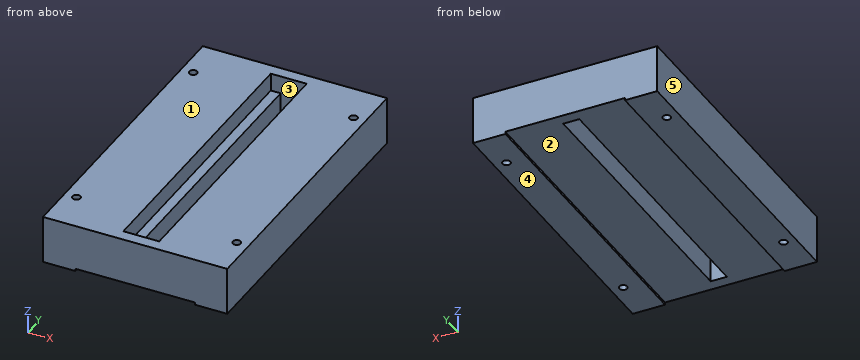
Autodesk Fusion 360 part; units mm, degrees
sketch "Sketch1" plane through (0, 0, 0) normal (0, 0, 1) x (1, 0, 0)
  line L0 (-38.5, 65) -> (38.5, 65)
  line L1 (38.5, 65) -> (38.5, -65)
  line L2 (38.5, -65) -> (-38.5, -65)
  line L3 (-38.5, -65) -> (-38.5, 65)
  line L4 (0, 65) -> (0, 0)
  line L5 (0, 0) -> (38.5, 0)
  line L6 (-33.5, -47.5) -> (-33.5, -65)
  line L7 (-33.5, -47.5) -> (-38.5, -47.5)
  line L8 (-33.5, 47.5) -> (-33.5, 65)
  line L9 (-33.5, 47.5) -> (-38.5, 47.5)
  line L10 (33.5, 47.5) -> (38.5, 47.5)
  line L11 (33.5, 47.5) -> (33.5, 65)
  line L12 (33.5, -47.5) -> (38.5, -47.5)
  line L13 (33.5, -47.5) -> (33.5, -65)
  point P0 (-33.5, 47.5)
  point P1 (33.5, 47.5)
  point P2 (33.5, -47.5)
  point P3 (-33.5, -47.5)
  dimension "d2" = 77
  dimension "d3" = 130
  dimension "d21" = 5
  dimension "d22" = 17.5
extrude "Extrude1" add sketch "Sketch1" along normal blind 20
hole "Hole1" at (-33.5, 47.5, 0) at (33.5, 47.5, 0) at (-33.5, -47.5, 0) at (33.5, -47.5, 0) direction (0, 0, 1) diameter 3.3 end through all
sketch "Sketch2" plane through (0, 0, 20) normal (0, 0, 1) x (-1, 0, 0)
  circle A0 centre (33.5, 47.5) radius 1.65
  circle A1 centre (33.5, -47.5) radius 1.65
  circle A2 centre (-33.5, -47.5) radius 1.65
  circle A3 centre (-33.5, 47.5) radius 1.65
  line L0 (38.5, 65) -> (-38.5, 65)
  line L1 (-38.5, 65) -> (-38.5, -65)
  line L2 (-38.5, -65) -> (38.5, -65)
  line L3 (38.5, -65) -> (38.5, 65)
  line L4 (0, 0) -> (-7.5, 0)
  line L5 (0, 0) -> (0, -60)
  line L6 (7.5, -60) -> (-7.5, -60)
  line L7 (-7.5, -60) -> (-7.5, 60)
  line L8 (-7.5, 60) -> (7.5, 60)
  line L9 (7.5, 60) -> (7.5, -60)
  dimension "d12" = 15
  dimension "d13" = 120
extrude "Extrude2" cut sketch "Sketch2" against normal blind 7.5 contours L4 L5 L6 L7 | L4 L5 L6 L7 L8 L9
sketch "Sketch3" plane through (0, 0, 12.5) normal (0, 0, 1) x (-1, 0, 0)
  line L0 (7.5, 60) -> (-7.5, 60)
  line L1 (-7.5, 60) -> (-7.5, -60)
  line L2 (-7.5, -60) -> (7.5, -60)
  line L3 (7.5, -60) -> (7.5, 60)
  line L4 (0, 0) -> (0, -60)
  line L5 (0, 0) -> (-3.375, 0)
  line L6 (3.375, -60) -> (-3.375, -60)
  line L7 (-3.375, -60) -> (-3.375, 60)
  line L8 (-3.375, 60) -> (3.375, 60)
  line L9 (3.375, 60) -> (3.375, -60)
  dimension "d16" = 120
  dimension "d17" = 6.75
extrude "Extrude3" cut sketch "Sketch3" against normal through all contours L0 L2 L4 L5 L6 L7 L8 L9 | L2 L4 L5 L6 L7
sketch "Sketch4" plane through (0, 0, 0) normal (0, 0, 1) x (1, 0, 0)
  line L0 (0, 0) -> (25, 0)
  line L1 (0, 0) -> (0, -65)
  line L2 (-25, -65) -> (25, -65)
  line L3 (25, -65) -> (25, 65)
  line L4 (25, 65) -> (-25, 65)
  line L5 (-25, 65) -> (-25, -65)
  dimension "d23" = 130
  dimension "d26" = 50
extrude "Extrude5" cut sketch "Sketch4" along normal blind 1
extrude "Extrude4" [suppressed]
Can you work these out from the model? Positions are in its coordinate system, mm. Face numbers are marked on the shaded views. A direction names the side the tool comes from. Round coordinates to 2 decimals unless told otherwise and drop trailing zeros. Loops run counter-clockwise (first coordinate to the right, second up) from the corner with the lowest first, then second, coordinate; pieces in that order, holes last. Notation, with made-up numbers: (-21.75, 58.5) -> (24.25, 58.5) arc R35 cw to (24.25, 96.5) -> close; hole circle Ø10 at (-27, 30). An arc over 180 degrees is marked (long way). Answer in a Markdown table with one row per item.
Item 1: We'd pull the mould along X, two halves only. Please class the marked faces 3, 4 and 5: released by +X, released by -X, zero draft, split by the parting line, or undercut.
Answer block:
| item | result |
|---|---|
| face 3 | undercut |
| face 4 | zero draft |
| face 5 | released by -X |
Item 2: Will these pins go through, and if not, where does the flat tip stop? P1, Ø1.5, axis at x = -10, y = 21.5, coming from the -Z side; P2, Ø2.5, axis at x = -33.5, y = 47.5, coming from the -Z side; P3, Ø1.2, axis at x = -5, y = -7, coming from the +Z side.
Answer block:
| item | result |
|---|---|
| P1 | z = 1 |
| P2 | through |
| P3 | z = 12.5 |
Item 3: On a 3-axis mill with a long thin cutter (end or side, diameter ignored), from which of +Z, -Z, +X, -X, +Y, -Y can I reach the whole of each face in a straight line? I mean the marked faces 1 and 2. Say none if no direction works.
Answer block:
| item | result |
|---|---|
| face 1 | +Z, +X, -X, +Y, -Y |
| face 2 | -Z, +Y, -Y |
Item 4: If I drill on probe 1 along X at (y, z) = (47.5, 9.25) (3 decimals); probe 2 along Y at (x, z) = (-33.5, 11); probe 3 along X at (y, z) = (-47.5, 13.25), over which ranges is the centre line in solid material (lowest first)?
Answer block:
| item | result |
|---|---|
| probe 1 | -38.5 to -35.15, -31.85 to -3.375, 3.375 to 31.85, 35.15 to 38.5 |
| probe 2 | -65 to -49.15, -45.85 to 45.85, 49.15 to 65 |
| probe 3 | -38.5 to -35.15, -31.85 to -7.5, 7.5 to 31.85, 35.15 to 38.5 |
Item 5: Suppose I cut it at B-B, the plane y = -1. List the corners of the cut face in (x, z) for me (3 decimals), plus the area to 3 significant figures.
Answer block:
| item | result |
|---|---|
| outline | (-38.5, 0) -> (-25, 0) -> (-25, 1) -> (-3.375, 1) -> (-3.375, 12.5) -> (-7.5, 12.5) -> (-7.5, 20) -> (-38.5, 20) -> close; (3.375, 1) -> (25, 1) -> (25, 0) -> (38.5, 0) -> (38.5, 20) -> (7.5, 20) -> (7.5, 12.5) -> (3.375, 12.5) -> close |
| area | 1,300 mm² |
Item 6: Suppose I cut it at C-C, the plane x = 33.5. List the corners of the cut face in (y, z) for me.
Answer block:
| item | result |
|---|---|
| outline | (-65, 0) -> (-49.15, 0) -> (-49.15, 20) -> (-65, 20) -> close; (-45.85, 0) -> (45.85, 0) -> (45.85, 20) -> (-45.85, 20) -> close; (49.15, 0) -> (65, 0) -> (65, 20) -> (49.15, 20) -> close |
Item 7: Suppose I cut it at D-D, the plane x = 0.5. List the corners of the cut face in (y, z) for me, plus the area to 3 significant figures.
Answer block:
| item | result |
|---|---|
| outline | (-65, 1) -> (-60, 1) -> (-60, 20) -> (-65, 20) -> close; (60, 1) -> (65, 1) -> (65, 20) -> (60, 20) -> close |
| area | 190 mm² |
Item 8: Suppose I cut it at A-A, the plane z = 8.75. List the corners of the cut face in (x, y) for me (3 decimals).
Answer block:
| item | result |
|---|---|
| outline | (-38.5, -65) -> (38.5, -65) -> (38.5, 65) -> (-38.5, 65) -> close; hole circle Ø3.3 at (-33.5, -47.5); hole circle Ø3.3 at (-33.5, 47.5); hole (-3.375, -60) -> (3.375, -60) -> (3.375, 60) -> (-3.375, 60) -> close; hole circle Ø3.3 at (33.5, -47.5); hole circle Ø3.3 at (33.5, 47.5) |
